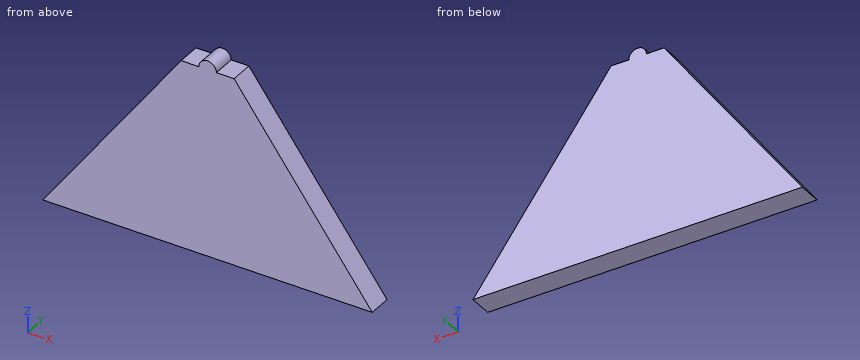
```python
from build123d import *

# Parameters (mm, degrees)
F1_DEPTH = 50.8


with BuildPart() as f1:
    # F0 (on Front) → F1 (new body)
    with BuildSketch(Plane.XZ):
        with BuildLine():
            Line((19.05, 63.5000025991), (0, 63.5000025991))
            Line((0, 63.5000025991), (-19.05, 63.5000025991))
            ThreePointArc((-19.05, 63.5000025991), (0, 44.4500025991), (19.05, 63.5000025991))
        make_face()
        with BuildLine():
            Line((-19.05, 63.5000025991), (0, 63.5000025991))
            Line((0, 63.5000025991), (19.05, 63.5000025991))
            ThreePointArc((19.05, 63.5000025991), (0, 82.5500025991), (-19.05, 63.5000025991))
        make_face()
        with BuildLine():
            ThreePointArc((19.05, 63.5000025991), (0, 44.4500025991), (-19.05, 63.5000025991))
            Line((-19.05, 63.5000025991), (-57.15, 63.5000025991))
            Line((-57.15, 63.5000025991), (-355.6, -342.8999974009))
            Line((-355.6, -342.8999974009), (0, -342.8999974009))
            Line((0, -342.8999974009), (57.15, -342.8999974009))
            Line((57.15, -342.8999974009), (57.15, 63.5000025991))
            Line((57.15, 63.5000025991), (19.05, 63.5000025991))
        make_face()
        Polygon((355.6, -342.8999974009), (57.15, 63.5000025991), (57.15, -342.8999974009), align=None)
    extrude(amount=F1_DEPTH)


solid = f1.part
```
Geometry: final body of the model. Coordinates: model frame, mm. Give positions to 0.01 mm unless a question says otherwise; leave off trailing zeros. Order: outer loops, then holes, each group sorted by start corner. A loop starts at its lowest first (then second) coordinate and runs counter-clockwise, first axis right, second up. Notation, with made-up numbers: M -26,1.25 L 17,1.25 A21 cw 17,17.25 Z; hole C -21,85 d1. An arc over 180 degrees is marked long. Answer as CSV lines item,"result". Start each with the question number.
1) First-contact query: P1, Ø1.5, axis at x = 45, y = -7, coming from the +Z side; P2, Ø6, axis at y = -38, z = -15, coming from the +X side; P3, Ø1, axis at x = 9, y = -23.5, coming from the +Z side. Flat tips, straight axial feed; report the tip coordinate or a pass-through.
2) Cut plane C-C (x = -297.5). Output: boundary loops of the cut face in (y, z).
3) Cut plane A-A (y = -39.5). Output: boundary loops of the cut face in (x, z), then the cut area to 3 significant figures.
4) Line query: line 1 (Z direction, x = -48, y = -24.5); line 2 (Z direction, x = -182.5, y = -30); line 3 (X direction, y = -32, z = -8.5) (3 decimals). Output: solid intervals per line, ascending. Write a range as from..to.
5) Cut plane B-B (z = -96.5). Output: boundary loops of the cut face in (x, y).
Findings below:
1,P1,"stops at z = 63.5"
1,P2,"stops at x = 117"
1,P3,"stops at z = 80.55"
2,outline,"M -50.8,-342.9 L 0,-342.9 L 0,-263.79 L -50.8,-263.79 Z"
3,outline,"M -355.6,-342.9 L 355.6,-342.9 L 57.15,63.5 L 19.05,63.5 A19.05 ccw -19.05,63.5 L -57.15,63.5 Z"
3,area,"168,000 mm²"
4,line 1,"z = -342.9..63.5"
4,line 2,"z = -342.9..-107.19"
4,line 3,"x = -110.025..110.025"
5,outline,"M -174.65,-50.8 L 174.65,-50.8 L 174.65,0 L -174.65,0 Z"
